```python
from build123d import *

# Parameters (mm, degrees)
F0_W     = 160
F0_H     = 20
F0_R     = 4
F0_W_2   = 50
F0_H_2   = 6.35
F1_DEPTH = 6.35


# Not quite as in the source:
# - a length typed as a fraction of an inch, garbled in the dataset ("3 / 203.2 mm" for 3/8 in), is restored


with BuildPart() as f1:
    # F0 (on Front) → F1 (new body)
    with BuildSketch(Plane.XZ):
        Rectangle(F0_W, F0_H)
        with Locations((-60, 0)):
            Circle(F0_R, mode=Mode.SUBTRACT)
        Rectangle(F0_W_2, F0_H_2, mode=Mode.SUBTRACT)
        with Locations((60, 0)):
            Circle(F0_R, mode=Mode.SUBTRACT)
    extrude(amount=F1_DEPTH)


solid = f1.part
```
Read the model definition and answer for the solid it produces. Units are mm, in the model's axes. A direction names the side the tool comes from. Give positions to 0.01 mm unless a question says otherwise; leave off trailing zeros. Order: outer loops, then holes, each group sorted by start corner. A loop starts at its lowest first (then second) coordinate and runs counter-clockwise, first axis right, second up.
(1) Given pin 1 (3 mm diameter, centred on x = 4, z = 0, fed in from +Y); pin 2 (6 mm diameter, centred on x = 27, z = -1, fed in from +Y), each flat-ended and moving along its own axis, determine where each tip first touches the part or whether it passes through.
(2) For a pull along Z with two mould halves and no side action, classify faces 3 (the flat face through (-1, -3, -10)), 4 (the flat face through (0, -3, 3.175)), 5 (the flat face through (-1, -3, 10)) as released by +Z, released by -Z, zero draft, split by the parting line, or undercut.
(3) Find section A-A (y = -1.5). Give the vertices of the cut face in (x, z) (3 decimals).
(4) Find section C-C (z = 0). Give the vertices of the cut face in (x, y), plus the area to 3 significant figures.
(5) Find section B-B (x = -60). Give the vertices of the cut face in (y, z), plus the area to 3 significant figures.
(6) For faces 1 (the flat face through (25, -3, 0)), 2 (the flat face through (-1, -6.35, 5)), determine the directions among +Z, -Z, +X, -X, +Y, -Y from which every point of the face is accessible in a straight line to the end or side of a thin tool.
(7) Find section D-D (x = -22). Give the vertices of the cut face in (y, z) (3 decimals).
(8) Straight lines are drawn through the part: L1, parallel to Z at x = 15, y = -3.25 (3 decimals); L2, parallel to X at y = -5.75, z = -2.25; L3, parallel to Z at x = 60, y = -2. For each, find the intervals that lie inside material, in ascending order.
Result sheet:
1. pin 1: passes through
1. pin 2: stops at y = 0
2. face 3: released by -Z
2. face 4: undercut
2. face 5: released by +Z
3. outline: (-80, -10) - (80, -10) - (80, 10) - (-80, 10) - close; hole circle Ø8 at (-60, 0); hole (-25, -3.175) - (25, -3.175) - (25, 3.175) - (-25, 3.175) - close; hole circle Ø8 at (60, 0)
4. outline: (-80, -6.35) - (-64, -6.35) - (-64, 0) - (-80, 0) - close; (-56, -6.35) - (-25, -6.35) - (-25, 0) - (-56, 0) - close; (25, -6.35) - (56, -6.35) - (56, 0) - (25, 0) - close; (64, -6.35) - (80, -6.35) - (80, 0) - (64, 0) - close
4. area: 597 mm2
5. outline: (-6.35, -10) - (0, -10) - (0, -4) - (-6.35, -4) - close; (-6.35, 4) - (0, 4) - (0, 10) - (-6.35, 10) - close
5. area: 76.2 mm2
6. face 1: +Y, -Y
6. face 2: +Z, -Z, +X, -X, -Y
7. outline: (-6.35, -10) - (0, -10) - (0, -3.175) - (-6.35, -3.175) - close; (-6.35, 3.175) - (0, 3.175) - (0, 10) - (-6.35, 10) - close
8. L1: z = -10 to -3.175, 3.175 to 10
8. L2: x = -80 to -63.31, -56.69 to -25, 25 to 56.69, 63.31 to 80
8. L3: z = -10 to -4, 4 to 10
